Model file for the job. Use its own axes, mm. A direction names the side the tool comes from. Round coordinates to 2 decimals unless told otherwise and drop trailing zeros. Loops run counter-clockwise (first coordinate to the right, second up) from the corner with the lowest first, then second, coordinate; pieces in that order, holes last. Notation, with made-up numbers: M 83,-8.5 L 94,-8.5 A25 ccw 94,15.5 Z; hole C 14,18 d4. An arc over 180 degrees is marked long. Use a Markdown table: item, result. Add a question column.
Q1. Cut at C-C (y = 3.5). Give the cut face in (x, z).
Q2. Probe line 1 (Z direction, x = 5, y = 4.25); line 2 (Z direction, x = -12.5, y = 2.5); line 3 (Y direction, x = -0.75, z = -26). List the from-to ranges inside material, lowest first. Write a range as from..to.
Q3. Cut at D-D (z = -7). Give the cut face in (x, y).
Q4. Tool access for faces 4 (the face through (0, 14.5, -17)), 5 (the face through (0.203, 17.735, -16.062)): list every direction of +Z, -Z, +X, -X, +Y, -Y with a clear straight run to the whole face (end or side of a thin tool).
Q5. Pin check, flat tips, straight feed: pin 1 (1.5 mm diameter, centred on x = 10.5, z = -23, fed in from -Y); pin 2 (4 mm diameter, centred on x = 4.5, y = 7, fed in from -Z); pin 3 (1.5 mm diameter, centred on x = 9, y = 13, fed in from +Z). Stop position of each tip, or through.
Q6. Cut at A-A (z = 1.5). Give the cut face in (x, y), plus the area to 3 significant figures.
Q7. Mould opens along Z. For faces 1 (the face through (-0.2, -0.09, -2.15)), 2 (the face through (0.2, 14.88, -29.56)), 3 (the face through (-0.203, 5.236, 2.466)) say: +Z half, -Z half, draft (parallel to the pull), parting line (faces both ways), or undercut.
Q8. Cut at B-B (y = -1.5). Give the cut face in (x, z), plus the area to 3 significant figures.
from build123d import *

# Parameters (mm, degrees)
SKETCH1_R           = 2.15
BOSS_EXTRUDE1_DEPTH = 14.5
FILLET1_R           = 2
FILLET2_R           = 1.4


with BuildPart() as part:
    # Sketch1 → Boss-Extrude1 (new, symmetric)
    with BuildSketch(Plane(origin=(0, 0, 0), x_dir=(0, 0, -1), z_dir=(1, 0, 0))):
        with BuildLine():
            Line((1.535973194, 18.500000001), (-2.572234834, 5.219922296))
            Line((-2.572234834, 5.219922296), (-1.768078738, 3.588021398))
            ThreePointArc((-1.768078738, 3.588021398), (-2.112780753, -3.396491935), (3.999999997, 1e-09))
            Line((3.999999997, 1e-09), (4.821445035, 14.000000001))
            Line((4.821445035, 14.000000001), (4.821445035, 14.500000001))
            Line((4.821445035, 14.500000001), (26.520495385, 14.500000001))
            Line((26.520495385, 14.500000001), (30.000000003, 14.500000001))
            Line((30.000000003, 14.500000001), (30.000000003, 17.000000001))
            Line((30.000000003, 17.000000001), (1.535973194, 18.500000001))
        make_face()
        with Locations(Location((0, 0, 0), (0, 0, 180))):
            Circle(SKETCH1_R, mode=Mode.SUBTRACT)
    extrude(amount=BOSS_EXTRUDE1_DEPTH, both=True)

    # Fillet1
    fillet1_edges = [part.edges().sort_by_distance(p)[0] for p in [
        (0, 18.500000001, -1.535973194),
    ]]
    fillet(fillet1_edges, radius=FILLET1_R)

    # Fillet2
    fillet2_edges = [part.edges().sort_by_distance(p)[0] for p in [
        (0, 3.588021398, 1.768078738),
        (0, 14.500000001, -4.821445035),
    ]]
    fillet(fillet2_edges, radius=FILLET2_R)
    # the kernel refuses this fillet: 1.4 mm, written as the material it takes off along each edge
    with BuildSketch(Plane(origin=(-15.893609334, 5.219922296, 2.572234834), x_dir=(0, -0.8970053501938902, -0.442019684769283), z_dir=(1, 0, 0))) as fillet2_2_piece_1:
        with BuildLine():
            CenterArc((FILLET2_R * 0.398174095356, FILLET2_R), FILLET2_R, 226.577668017, 43.422331983)
            Line((-FILLET2_R * 0.289196557818, FILLET2_R * 0.273693188002), (-FILLET2_R * 0.302943970882, FILLET2_R * 0.259167051762))
            Line((-FILLET2_R * 0.302943970882, FILLET2_R * 0.259167051762), (-FILLET2_R * 0.00796348190712, -FILLET2_R * 0.02))
            Line((-FILLET2_R * 0.00796348190712, -FILLET2_R * 0.02), (FILLET2_R * 0.398174095356, -FILLET2_R * 0.02))
            Line((FILLET2_R * 0.398174095356, -FILLET2_R * 0.02), (FILLET2_R * 0.398174095356, 0))
        make_face()
    extrude(amount=31.787218667, mode=Mode.SUBTRACT)
    with BuildSketch(Plane(origin=(17.820413203, 17.000000001, -30.000000003), x_dir=(0, 0.05262507378866547, 0.9986143407786299), z_dir=(-1, 0, 0))) as fillet2_2_piece_2:
        with BuildLine():
            CenterArc((FILLET2_R * 0.948689486547, -FILLET2_R), FILLET2_R, 90, 86.983411926)
            Line((-FILLET2_R * 0.049924854232, -FILLET2_R * 0.947374926211), (-FILLET2_R * 0.0698971410476, -FILLET2_R * 0.946322424736))
            Line((-FILLET2_R * 0.0698971410476, -FILLET2_R * 0.946322424736), (-FILLET2_R * 0.0189737897309, FILLET2_R * 0.02))
            Line((-FILLET2_R * 0.0189737897309, FILLET2_R * 0.02), (FILLET2_R * 0.948689486547, FILLET2_R * 0.02))
            Line((FILLET2_R * 0.948689486547, FILLET2_R * 0.02), (FILLET2_R * 0.948689486547, 0))
        make_face()
    extrude(amount=35.640826406, mode=Mode.SUBTRACT)
    with BuildSketch(Plane(origin=(18, 14.500000001, -30.000000003), x_dir=(0, 1, 0), z_dir=(-1, 0, 0))) as fillet2_2_piece_3:
        with BuildLine():
            CenterArc((FILLET2_R, -FILLET2_R), FILLET2_R, 90, 90)
            Line((0, -FILLET2_R), (-FILLET2_R * 0.02, -FILLET2_R))
            Line((-FILLET2_R * 0.02, -FILLET2_R), (-FILLET2_R * 0.02, FILLET2_R * 0.02))
            Line((-FILLET2_R * 0.02, FILLET2_R * 0.02), (FILLET2_R, FILLET2_R * 0.02))
            Line((FILLET2_R, FILLET2_R * 0.02), (FILLET2_R, 0))
        make_face()
    extrude(amount=36, mode=Mode.SUBTRACT)


solid = part.part
Checked values:
| question | item | result |
|---|---|---|
| 1 | outline | M -14.5,-4.21 L 14.5,-4.21 L 14.5,2.28 L -14.5,2.28 Z |
| 2 | line 1 | z = -4.25..2.17 |
| 2 | line 2 | z = -4.15..3.12 |
| 2 | line 3 | y = 14.5..17.21 |
| 3 | outline | M -14.5,14.5 L 14.5,14.5 L 14.5,18.21 L -14.5,18.21 Z |
| 4 | face 4 | -Z, +X, -X, -Y |
| 4 | face 5 | -Z, +X, -X, +Y |
| 5 | pin 1 | stops at y = 14.5 |
| 5 | pin 2 | stops at z = -4.53 |
| 5 | pin 3 | stops at z = 0.4 |
| 6 | outline | M -14.5,-3.71 L 14.5,-3.71 L 14.5,-1.54 L -14.5,-1.54 Z; M -14.5,1.54 L 14.5,1.54 L 14.5,8.69 L -14.5,8.69 Z |
| 6 | area | 270 mm^2 |
| 7 | face 1 | undercut |
| 7 | face 2 | -Z half |
| 7 | face 3 | +Z half |
| 8 | outline | M -14.5,-3.71 L 14.5,-3.71 L 14.5,-1.54 L -14.5,-1.54 Z; M -14.5,1.54 L 14.5,1.54 L 14.5,3.71 L -14.5,3.71 Z |
| 8 | area | 126 mm^2 |
